Part print with two shaded views. Sizes in mm from the minimum x, y, z corner. A direction names the side the tool comes from. Coordinates: 2 decimals unless noted, no trailing zeros. Order: outer loops, then holes, each group sorted by start corner. A loop starts at its lowest first (then second) coordinate and runs counter-clockwise, first axis right, second up. Notation, with made-up numbers: (80.5, 9) - (135.5, 9) arc R23 cw to (135.5, 20) - close; hole circle Ø6 at (6, 21). An arc over 180 degrees is marked (long way). Write each question's results on one line, items separated by ' | '. Start each with the question number.
Q1. Band-saw the part on A-A, the plane z = 52.5. Write the cut outline in (x, y), then the cut area to 3 significant figures.
Q2. Pin check, flat tips, straight feed: P1, Ø12, axis at x = 46, y = 102, coming from the +Z side; P2, Ø5, axis at y = 185, z = 110, coming from the -X side; P3, Ø4, axis at x = 25, z = 146, coming from the -Y side. Stop position of each tip, or through.
Q3. Band-saw the part on B-B, the plane x = 23. Write the cut outline in (y, z).
Q4. Wall check: probe 1 along Z at (x, y) = (19, 186); probe 2 along Z at (x, y) = (27, 10); probe 3 along Y at (x, z) = (53.5, 12). Give the ranges that are in metal, low to high.
Q5. Which spindle directions (+Z, -Z, +X, -X, +Y, -Y) get a long thin tool onto all of the face, cutting with end or side? Do the marked faces 1, 2 and 3. Say none if no direction does.
Q6. Band-saw the part on C-C, the plane z = 26. Write the cut outline in (x, y).
Q7. Band-saw the part on D-D, the plane y = 140.5. Write the cut outline in (x, z), then the cut area to 3 significant figures.
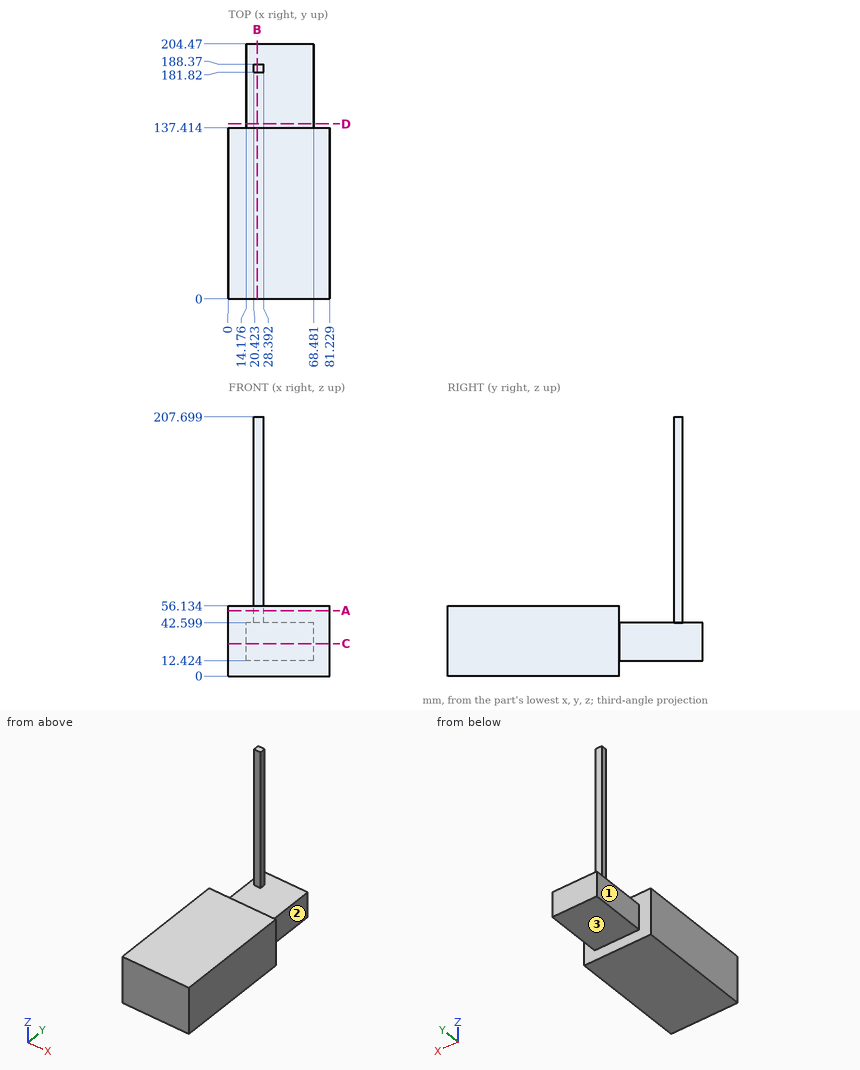
Results below:
1) outline: (0, 0) - (81.23, 0) - (81.23, 137.41) - (0, 137.41) - close; (20.42, 181.82) - (28.39, 181.82) - (28.39, 188.37) - (20.42, 188.37) - close | area: 11,200 mm²
2) P1: stops at z = 56.13 | P2: stops at x = 20.42 | P3: stops at y = 181.82
3) outline: (0, 0) - (137.41, 0) - (137.41, 12.42) - (204.47, 12.42) - (204.47, 42.6) - (188.37, 42.6) - (188.37, 207.7) - (181.82, 207.7) - (181.82, 42.6) - (137.41, 42.6) - (137.41, 56.13) - (0, 56.13) - close
4) probe 1: z = 12.42 to 42.6 | probe 2: z = 0 to 56.13 | probe 3: y = 0 to 137.41
5) face 1: +Z, -Z, -X, +Y | face 2: +Z, -Z, +X, +Y | face 3: -Z, +X, -X, +Y
6) outline: (0, 0) - (81.23, 0) - (81.23, 137.41) - (68.48, 137.41) - (68.48, 204.47) - (14.18, 204.47) - (14.18, 137.41) - (0, 137.41) - close
7) outline: (14.18, 12.42) - (68.48, 12.42) - (68.48, 42.6) - (14.18, 42.6) - close | area: 1,640 mm²
